```python
from build123d import *

# Parameters (mm, degrees)
CROQUIS1_W                   = 356
CROQUIS1_H                   = 456
SALIENTE_EXTRUIR1_DEPTH      = 160
REDONDEO1_R                  = 10
CORTAR_EXTRUIR1_DEPTH        = 2.5
CORTAR_EXTRUIR1_DEPTH_BACK   = 2.5
CORTAR_EXTRUIR1_START        = -25
CROQUIS2_W                   = 356
CROQUIS2_H                   = 456
CROQUIS2_W_2                 = 336
CROQUIS2_H_2                 = 436
REDONDEO2_R                  = 10
SALIENTE_EXTRUIR2_DEPTH      = 5
SALIENTE_EXTRUIR2_DEPTH_BACK = 5
REDONDEO6_R                  = 3
REDONDEO7_R                  = 3
REDONDEO8_R                  = 3
CROQUIS5_W                   = 32.5
CROQUIS5_H                   = 24.2
CROQUIS5_H_2                 = 24.275971101
CROQUIS5_H_3                 = 24.099571128
CROQUIS5_H_4                 = 23.966296081
CORTAR_EXTRUIR2_DEPTH        = 20


# Some blends are built 0.0001 mm under size
with BuildPart() as part:
    # Croquis1 → Saliente-Extruir1 (new body)
    with BuildSketch(Plane.XY):
        Rectangle(CROQUIS1_W, CROQUIS1_H)
    extrude(amount=SALIENTE_EXTRUIR1_DEPTH)

    # Redondeo1
    redondeo1_edges = [part.edges().sort_by_distance(p)[0] for p in [
        (-178, 0, 160),
        (0, -228, 160),
        (178, 0, 160),
        (178, -228, 80),
        (-178, -228, 80),
        (-178, 228, 80),
        (178, 228, 80),
        (0, 228, 160),
    ]]
    fillet(redondeo1_edges, radius=REDONDEO1_R)

    # Croquis2 → Cortar-Extruir1 (cut, two sides: drawn at the far end of the back side and taken through both)
    with BuildSketch(Plane.XY.offset(160).offset(CORTAR_EXTRUIR1_START - CORTAR_EXTRUIR1_DEPTH_BACK)):
        Rectangle(CROQUIS2_W, CROQUIS2_H)
        Rectangle(CROQUIS2_W_2, CROQUIS2_H_2, mode=Mode.SUBTRACT)
    extrude(amount=CORTAR_EXTRUIR1_DEPTH + CORTAR_EXTRUIR1_DEPTH_BACK, mode=Mode.SUBTRACT)

    # Redondeo2
    redondeo2_edges = [part.edges().sort_by_distance(p)[0] for p in [
        (168, 218, 135),
        (-168, 218, 135),
        (-168, -218, 135),
        (168, -218, 135),
    ]]
    fillet(redondeo2_edges, radius=REDONDEO2_R)

    # Croquis4 → Saliente-Extruir2 (add, two sides: drawn at the far end of the back side and taken through both)
    with BuildSketch(Plane.XY.offset(65).offset(-SALIENTE_EXTRUIR2_DEPTH_BACK)):
        with BuildLine():
            Line((168, -231), (-168, -231))
            ThreePointArc((-168, -231), (-177.192388155, -227.192388155), (-181, -218))
            Line((-181, -218), (-181, 218))
            ThreePointArc((-181, 218), (-177.192388155, 227.192388155), (-168, 231))
            Line((-168, 231), (168, 231))
            ThreePointArc((168, 231), (177.192388155, 227.192388155), (181, 218))
            Line((181, 218), (181, -218))
            ThreePointArc((181, -218), (177.192388155, -227.192388155), (168, -231))
        make_face()
    extrude(amount=SALIENTE_EXTRUIR2_DEPTH + SALIENTE_EXTRUIR2_DEPTH_BACK)

    # Redondeo6
    redondeo6_edges = [part.edges().sort_by_distance(p)[0] for p in [
        (-177.192388155, 227.192388155, 70),
        (-181, 0, 70),
        (-177.192388155, -227.192388155, 70),
        (0, -231, 70),
        (177.192388155, -227.192388155, 70),
        (181, 0, 70),
        (177.192388155, 227.192388155, 70),
        (0, 231, 70),
        (-177.192388155, 227.192388155, 60),
        (0, 231, 60),
        (177.192388155, 227.192388155, 60),
        (181, 0, 60),
        (177.192388155, -227.192388155, 60),
        (0, -231, 60),
        (-177.192388155, -227.192388155, 60),
        (-181, 0, 60),
    ]]
    fillet(redondeo6_edges, radius=REDONDEO6_R - 0.0001)  # a hair under: the kernel refuses the full size

    # Redondeo7
    # the kernel refuses this fillet: 3 mm, written as the material it adds along each edge
    with BuildSketch(Plane(origin=(178, 218, 60), x_dir=(0.9659313848535178, 0, 0.25879829936644666), z_dir=(0, -1, 0)), Plane(origin=(-178, -218, 60), x_dir=(-0.9659313848535145, 0, 0.25879829936645976), z_dir=(0, 1, 0))) as redondeo7_piece_1:
        with BuildLine():
            CenterArc((2.329422704, -2.897768274), REDONDEO7_R, 105.000679234, 60.000551337)
            Line((-0.56837145, -2.121373376), (-0.858150866, -2.043733886))
            Line((-0.858150866, -2.043733886), (-0.289779415, 0.07763949))
            Line((-0.289779415, 0.07763949), (0.07763949, 0.289779415))
            ThreePointArc((0.07763949, 0.289779415), (0.077736083, 0.289753536), (1.475282068, 0.289776827))
            Line((1.475282068, 0.289776827), (1.552931216, 0))
        make_face()
    extrude(amount=436)
    with BuildSketch(Plane(origin=(-168, -218, 60), x_dir=(-1, 0, 0), z_dir=(0, 1, 0))) as redondeo7_piece_2:
        with BuildLine():
            CenterArc((13, -2.196194687), REDONDEO7_R, 119.999448663, 60.000551337)
            Line((10, -2.196194687), (9.7, -2.196194687))
            Line((9.7, -2.196194687), (9.7, 0))
            Line((9.7, 0), (10, 0.3))
            ThreePointArc((10, 0.3), (10.0001, 0.3), (11.3500275, 0.661705022))
            Line((11.3500275, 0.661705022), (11.500025, 0.401895958))
        make_face()
    revolve(axis=Axis((-168, -218, 60), (0, 0, 1)), revolution_arc=90)
    with BuildSketch(Plane(origin=(168, -218, 60), x_dir=(0, -1, 0), z_dir=(-1, 0, 0))) as redondeo7_piece_3:
        with BuildLine():
            CenterArc((13, -2.196194687), REDONDEO7_R, 119.999448663, 60.000551337)
            Line((10, -2.196194687), (9.7, -2.196194687))
            Line((9.7, -2.196194687), (9.7, 0))
            Line((9.7, 0), (10, 0.3))
            ThreePointArc((10, 0.3), (10.0001, 0.3), (11.3500275, 0.661705022))
            Line((11.3500275, 0.661705022), (11.500025, 0.401895958))
        make_face()
    revolve(axis=Axis((168, -218, 60), (0, 0, 1)), revolution_arc=90)
    with BuildSketch(Plane(origin=(168, 218, 60), x_dir=(1, 0, 0), z_dir=(0, -1, 0))) as redondeo7_piece_4:
        with BuildLine():
            CenterArc((13, -2.196194687), REDONDEO7_R, 119.999448663, 60.000551337)
            Line((10, -2.196194687), (9.7, -2.196194687))
            Line((9.7, -2.196194687), (9.7, 0))
            Line((9.7, 0), (10, 0.3))
            ThreePointArc((10, 0.3), (10.0001, 0.3), (11.3500275, 0.661705022))
            Line((11.3500275, 0.661705022), (11.500025, 0.401895958))
        make_face()
    revolve(axis=Axis((168, 218, 60), (0, 0, 1)), revolution_arc=90)
    with BuildSketch(Plane(origin=(-168, 218, 60), x_dir=(0, 1, 0), z_dir=(1, 0, 0))) as redondeo7_piece_5:
        with BuildLine():
            CenterArc((13, -2.196194687), REDONDEO7_R, 119.999448663, 60.000551337)
            Line((10, -2.196194687), (9.7, -2.196194687))
            Line((9.7, -2.196194687), (9.7, 0))
            Line((9.7, 0), (10, 0.3))
            ThreePointArc((10, 0.3), (10.0001, 0.3), (11.3500275, 0.661705022))
            Line((11.3500275, 0.661705022), (11.500025, 0.401895958))
        make_face()
    revolve(axis=Axis((-168, 218, 60), (0, 0, 1)), revolution_arc=90)
    with BuildSketch(Plane(origin=(-168, 228, 60), x_dir=(0, 0.9659313848535145, 0.25879829936645976), z_dir=(1, 0, 0)), Plane(origin=(168, -228, 60), x_dir=(0, -0.9659313848535215, 0.2587982993664339), z_dir=(-1, 0, 0))) as redondeo7_piece_6:
        with BuildLine():
            CenterArc((2.329422704, -2.897768274), REDONDEO7_R, 105.000679234, 60.000551337)
            Line((-0.56837145, -2.121373376), (-0.858150866, -2.043733886))
            Line((-0.858150866, -2.043733886), (-0.289779415, 0.07763949))
            Line((-0.289779415, 0.07763949), (0.07763949, 0.289779415))
            ThreePointArc((0.07763949, 0.289779415), (0.077736083, 0.289753536), (1.475282068, 0.289776827))
            Line((1.475282068, 0.289776827), (1.552931216, 0))
        make_face()
    extrude(amount=336)

    # Redondeo8
    # the kernel refuses this fillet: 3 mm, written as the material it adds along each edge
    with BuildSketch(Plane(origin=(178, 218, 70), x_dir=(0.965931384853519, 0, -0.2587982993664427), z_dir=(0, -1, 0)), Plane(origin=(-178, -218, 70), x_dir=(-0.9659313848535145, 0, -0.25879829936645976), z_dir=(0, 1, 0))) as redondeo8_piece_1:
        with BuildLine():
            CenterArc((2.329422704, 2.897768274), REDONDEO8_R, 194.99876943, 60.000551337)
            Line((-0.56837145, 2.121373376), (-0.858150866, 2.043733886))
            Line((-0.858150866, 2.043733886), (-0.289779415, -0.07763949))
            Line((-0.289779415, -0.07763949), (0.07763949, -0.289779415))
            ThreePointArc((0.07763949, -0.289779415), (0.077736083, -0.289753536), (1.475282068, -0.289776827))
            Line((1.475282068, -0.289776827), (1.552931216, 0))
        make_face()
    extrude(amount=436)
    with BuildSketch(Plane(origin=(-168, 228, 70), x_dir=(0, 0.9659313848535145, -0.25879829936645976), z_dir=(1, 0, 0)), Plane(origin=(168, -228, 70), x_dir=(0, -0.9659313848535178, -0.25879829936644666), z_dir=(-1, 0, 0))) as redondeo8_piece_2:
        with BuildLine():
            CenterArc((2.329422704, 2.897768274), REDONDEO8_R, 194.99876943, 60.000551337)
            Line((-0.56837145, 2.121373376), (-0.858150866, 2.043733886))
            Line((-0.858150866, 2.043733886), (-0.289779415, -0.07763949))
            Line((-0.289779415, -0.07763949), (0.07763949, -0.289779415))
            ThreePointArc((0.07763949, -0.289779415), (0.077736083, -0.289753536), (1.475282068, -0.289776827))
            Line((1.475282068, -0.289776827), (1.552931216, 0))
        make_face()
    extrude(amount=336)
    with BuildSketch(Plane(origin=(-168, -218, 70), x_dir=(-1, 0, 0), z_dir=(0, 1, 0))) as redondeo8_piece_3:
        with BuildLine():
            CenterArc((13, 2.196194687), REDONDEO8_R, 180, 60.000551337)
            Line((10, 2.196194687), (9.7, 2.196194687))
            Line((9.7, 2.196194687), (9.7, 0))
            Line((9.7, 0), (10, -0.3))
            ThreePointArc((10, -0.3), (10.0001, -0.3), (11.3500275, -0.661705022))
            Line((11.3500275, -0.661705022), (11.500025, -0.401895958))
        make_face()
    revolve(axis=Axis((-168, -218, 70), (0, 0, 1)), revolution_arc=90)
    with BuildSketch(Plane(origin=(168, -218, 70), x_dir=(0, -1, 0), z_dir=(-1, 0, 0))) as redondeo8_piece_4:
        with BuildLine():
            CenterArc((13, 2.196194687), REDONDEO8_R, 180, 60.000551337)
            Line((10, 2.196194687), (9.7, 2.196194687))
            Line((9.7, 2.196194687), (9.7, 0))
            Line((9.7, 0), (10, -0.3))
            ThreePointArc((10, -0.3), (10.0001, -0.3), (11.3500275, -0.661705022))
            Line((11.3500275, -0.661705022), (11.500025, -0.401895958))
        make_face()
    revolve(axis=Axis((168, -218, 70), (0, 0, 1)), revolution_arc=90)
    with BuildSketch(Plane(origin=(168, 218, 70), x_dir=(1, 0, 0), z_dir=(0, -1, 0))) as redondeo8_piece_5:
        with BuildLine():
            CenterArc((13, 2.196194687), REDONDEO8_R, 180, 60.000551337)
            Line((10, 2.196194687), (9.7, 2.196194687))
            Line((9.7, 2.196194687), (9.7, 0))
            Line((9.7, 0), (10, -0.3))
            ThreePointArc((10, -0.3), (10.0001, -0.3), (11.3500275, -0.661705022))
            Line((11.3500275, -0.661705022), (11.500025, -0.401895958))
        make_face()
    revolve(axis=Axis((168, 218, 70), (0, 0, 1)), revolution_arc=90)
    with BuildSketch(Plane(origin=(-168, 218, 70), x_dir=(0, 1, 0), z_dir=(1, 0, 0))) as redondeo8_piece_6:
        with BuildLine():
            CenterArc((13, 2.196194687), REDONDEO8_R, 180, 60.000551337)
            Line((10, 2.196194687), (9.7, 2.196194687))
            Line((9.7, 2.196194687), (9.7, 0))
            Line((9.7, 0), (10, -0.3))
            ThreePointArc((10, -0.3), (10.0001, -0.3), (11.3500275, -0.661705022))
            Line((11.3500275, -0.661705022), (11.500025, -0.401895958))
        make_face()
    revolve(axis=Axis((-168, 218, 70), (0, 0, 1)), revolution_arc=90)

    # Croquis5 → Cortar-Extruir2 (cut)
    with BuildSketch(Plane(origin=(178, 0, 0), x_dir=(0, 0, -1), z_dir=(1, 0, 0))):
        with Locations((-29.303847577, -154.422503433)):
            Rectangle(CROQUIS5_W, CROQUIS5_H)
        with Locations((-29.303847577, -121.606769627)):
            Rectangle(CROQUIS5_W, CROQUIS5_H_2)
        with Locations((-29.303847577, -76.907454446)):
            Rectangle(CROQUIS5_W, CROQUIS5_H_3)
        with Locations((-29.303847577, 76.415754786)):
            Rectangle(CROQUIS5_W, CROQUIS5_H_4)
    extrude(amount=-CORTAR_EXTRUIR2_DEPTH, mode=Mode.SUBTRACT)


solid = part.part
```
Geometry check sheet. Reference: the model listing, model coordinates, mm. A direction names the side the tool comes from. Coordinates: 2 decimals unless noted, no trailing zeros. Order: outer loops, then holes, each group sorted by start corner. A loop starts at its lowest first (then second) coordinate and runs counter-clockwise, first axis right, second up. Notation, with made-up numbers: (61.25, 56) - (83.25, 56) arc R13 cw to (83.25, 75) - close; hole circle Ø4 at (76, 46). An arc over 180 degrees is marked (long way). Answer in a Markdown table with one row per item. Add a question column.
1. Gauge pin test, flat ends, axial feed: pin 1 Ø2 at (y, z) = (-72.5, 72) entering from +X; pin 2 Ø1.5 at (x, z) = (-113, 104) entering from -Y; pin 3 Ø6 at (y, z) = (-139, 39) entering from -X. Record the tip position at first contact, or that the pin passes through.
2. Section check B-B (z = 21). Enter the section's corners in (x, y), plus the area to 3 significant figures.
3. Draft check along Z on faces 6 (the face through (175.15, 3.05, 156.99)), 7 (the face through (-165.15, 214.99, 135.04)), 8 (the face through (177.293, -227.091, 64.972)). Enter one of: +Z half, -Z half, draft (parallel to the pull), parting line (faces both ways), or undercut.
4. Material ranges on L1, parallel to X at y = -147.5, z = 90.5; L2, parallel to Y at x = -151, z = 39.5; L3, parallel to X at y = -165.5, z = 134, recorded low to high. Write a range as [from, to].
5. Access from +Z, -Z, +X, -X, +Y, -Y to the whole of each face (thin tool, end or side, straight path). Record for faces 1 (the face through (-175.15, -224.99, 143.84)), 2 (the face through (-175.15, -224.99, 29.31)), 3 (the face through (158, 77, 30)), 4 (the face through (175.15, 224.99, 29.31)), 5 (the face through (-2, 228, 28)).
6. Section check D-D (z = 115). Enter the section's corners in (x, y).
7. Section check C-C (y = 145.5). Enter the section's corners in (x, z), plus the area to 3 significant figures.
Data:
| question | item | result |
|---|---|---|
| 1 | pin 1 | stops at x = 178.25 |
| 1 | pin 2 | stops at y = -228 |
| 1 | pin 3 | stops at x = -178 |
| 2 | outline | (-178, -218) arc R10 ccw to (-168, -228) - (168, -228) arc R10 ccw to (178, -218) - (178, -166.52) - (158, -166.52) - (158, -142.32) - (178, -142.32) - (178, -133.74) - (158, -133.74) - (158, -109.47) - (178, -109.47) - (178, -88.96) - (158, -88.96) - (158, -64.86) - (178, -64.86) - (178, 64.43) - (158, 64.43) - (158, 88.4) - (178, 88.4) - (178, 218) arc R10 ccw to (168, 228) - (-168, 228) arc R10 ccw to (-178, 218) - close |
| 2 | area | 160,000 mm² |
| 3 | face 6 | +Z half |
| 3 | face 7 | undercut |
| 3 | face 8 | draft |
| 4 | L1 | x = [-178, 178] |
| 4 | L2 | y = [-228, 228] |
| 4 | L3 | x = [-168, 168] |
| 5 | face 1 | +Z, -X, -Y |
| 5 | face 2 | -Z, -X, -Y |
| 5 | face 3 | +X |
| 5 | face 4 | -Z, +X, +Y |
| 5 | face 5 | -Z, +X, -X, +Y |
| 6 | outline | (-178, -218) arc R10 ccw to (-168, -228) - (168, -228) arc R10 ccw to (178, -218) - (178, 218) arc R10 ccw to (168, 228) - (-168, 228) arc R10 ccw to (-178, 218) - close |
| 7 | outline | (-181, 63) arc R3 ccw to (-179.5, 60.4) arc R3 cw to (-178, 57.8) - (-178, 0) - (178, 0) - (178, 57.8) arc R3 cw to (179.5, 60.4) arc R3 ccw to (181, 63) - (181, 67) arc R3 ccw to (179.5, 69.6) arc R3 cw to (178, 72.2) - (178, 132.5) - (168, 132.5) - (168, 137.5) - (178, 137.5) - (178, 150) arc R10 ccw to (168, 160) - (-168, 160) arc R10 ccw to (-178, 150) - (-178, 137.5) - (-168, 137.5) - (-168, 132.5) - (-178, 132.5) - (-178, 72.2) arc R3 cw to (-179.5, 69.6) arc R3 ccw to (-181, 67) - close |
| 7 | area | 56,900 mm² |
